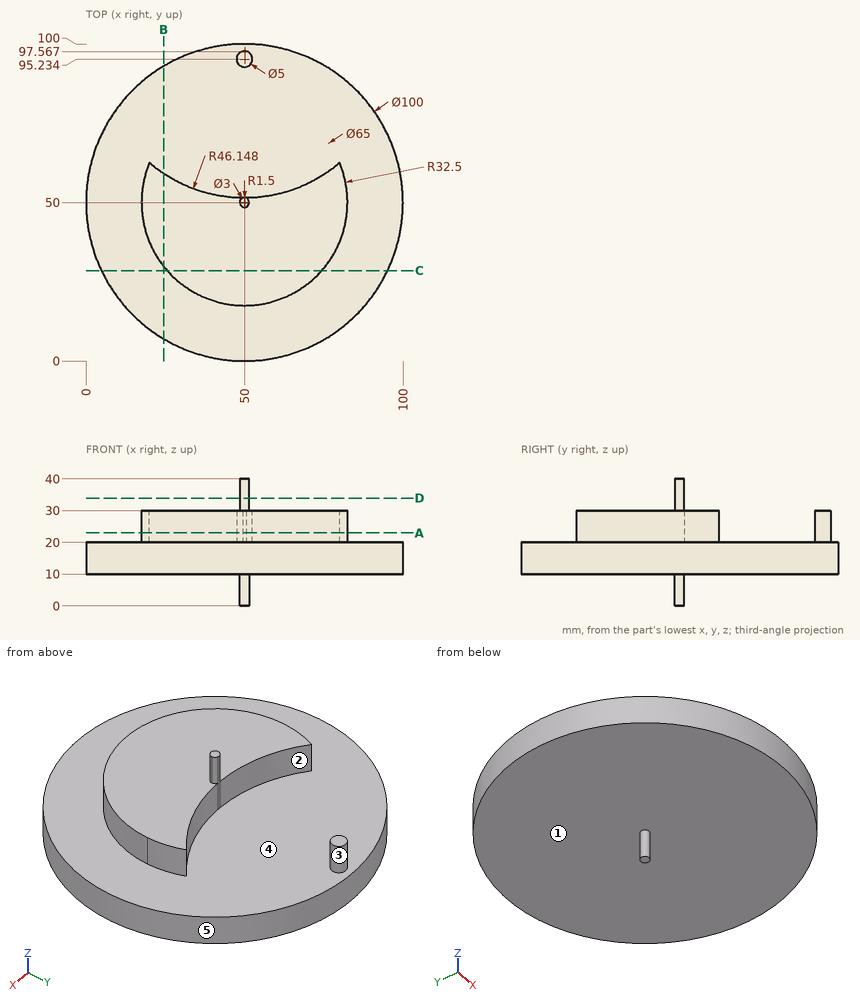
Answer from the drawing. Dimensions are ordinates in mm from the lowest x, y and z of the part. A direction names the side the tool comes from. Give positions to 0.01 mm unless a question says otherwise; leave off trailing zeros. Order: outer loops, then holes, each group sorted by start corner. A loop starts at its lowest first (then second) coordinate and runs counter-clockwise, first axis right, second up. Notation, with made-up numbers: (13, 68) -> (22, 68) arc R15 cw to (22, 90) -> close; hole circle Ø2 at (32, 22). An arc over 180 degrees is marked (long way). One line per item, written item: value. Start each with the question number.
(1) The part is cut by section D-D (z = 34). Determine the outline of the cut face in (x, y).
(2) For a pull along X with two mould halves and no side action, classify the marked faces 1, 2 and 3 as released by +X, released by -X, zero draft, split by the parting line, or undercut.
(3) Straight lines are drawn through the part: L1, parallel to Z at x = 67.5, y = 24.5; L2, parallel to Z at x = 56, y = 12; L3, parallel to X at y = 25, z = 23 (1 decimal). For each, find the intervals that lie inside material, in ascending order.
(4) Flat-ended cylindrical pins translate along their axes: P1, Ø2.5, axis at x = 50.5, y = 95.5, coming from the +Z side; P2, Ø1.5, axis at x = 59, y = 14, coming from the -Z side; P3, Ø4, axis at y = 10, z = 21, coming from the +X side; P4, Ø1, axis at y = 58.5, z = 32, coming from the -X side. Find the tip coordinate at first contact, or state that the pin passes through.
(5) A tool of negligible diameter and unlimited length cuts with its end or side. For the marked faces 4 and 5, from which of +Z, -Z, +X, -X, +Y, -Y can it reach the whole face along a straight path? Write none if from no direction.
(6) The part is cut by section A-A (z = 23). Determine the outline of the cut face in (x, y), and give its area (3 significant figures).
(7) The part is cut by section C-C (y = 28.5). Determine the outline of the cut face in (x, z).
(8) The part is cut by section B-B (x = 24.5). Determine the outline of the cut face in (y, z).
Taken from the geometry:
1. outline: circle Ø3 at (50, 50)
2. face 1: zero draft
2. face 2: undercut
2. face 3: split by the parting line
3. L1: 10 to 30
3. L2: 10 to 20
3. L3: 29.2 to 70.8
4. P1: z = 30
4. P2: z = 10
4. P3: x = 82.18
4. P4: through
5. face 4: +Z
5. face 5: +Z, -Z
6. outline: (20, 62.5) arc R32.5 ccw (long way) to (80, 62.5) arc R46.15 cw to (50.48, 51.42) arc R1.5 ccw to (49.52, 51.42) arc R46.15 cw to start; circle Ø5 at (50, 95.23)
6. area: 2,020 mm^2
7. outline: (4.86, 10) -> (95.14, 10) -> (95.14, 20) -> (74.37, 20) -> (74.37, 30) -> (25.63, 30) -> (25.63, 20) -> (4.86, 20) -> close
8. outline: (6.99, 10) -> (93.01, 10) -> (93.01, 20) -> (59.1, 20) -> (59.1, 30) -> (29.85, 30) -> (29.85, 20) -> (6.99, 20) -> close
